The figure shows three views and two pictorial views of one solid part (mm, origin at its lowest corner). Answer the questions. A direction names the side the tool comes from. Round coordinates to 2 decimals unless told otherwise and drop trailing zeros. Write each loop counter-clockwise with the first axis right and the second up, starting at its lowest first coordinate (ties: lowest second). Pieces come first, ordered by that corner, then holes. Notation, with made-up numbers: (2, 83.25) - (20, 83.25) arc R26 cw to (20, 106.25) - close; hole circle Ø5 at (-39, 37.5). An arc over 180 degrees is marked (long way). Answer as CSV lines item,"result". Start each with the question number.
Item 1: A cutting plane is placed at C-C on y = 8. Determine the outline of the cut face in (x, z), and give its area (3 significant figures).
Item 2: A cutting plane is placed at D-D on x = 132.5. Determine the outline of the cut face in (y, z).
Item 3: Flat-ended cylindrical pins translate along their axes: pin 1 (6 mm diameter, centred on y = 11.5, z = 10, fed in from +X); pin 2 (9 mm diameter, centred on x = 10, y = 17.5, fed in from +Z); pin 3 (10.5 mm diameter, centred on x = 98.5, y = 23, fed in from -Z). Find the tip coordinate at first contact, or state that the pin passes through.
Item 4: A cutting plane is placed at B-B on z = 24. Determine the outline of the cut face in (x, y), and give its area (3 significant figures).
Item 5: A cutting plane is placed at A-A on x = 220. Determine the outline of the cut face in (y, z).
Item 6: For a pull along X with two mould halves and no side action, classify the marked faces 1, 2 and 3 as pulls with the +X half, pulls with the -X half, needs draft (parallel to the pull), parting line crosses it, or undercut.
Item 7: Which of the six approach directions +Z, -Z, +X, -X, +Y, -Y give full straight-line access (tool end or side, diameter ignored) to the marked faces 4 and 5?
Item 8: Straight lines are drawn through the part: line 1 along X through (y, z) = (27, 6.5); line 2 along Y through (x, z) = (147.5, 48.6); line 3 along Y through (x, z) = (10, 1.1). For each, find the intervals that lie inside material, in ascending order. Write a range as [from, to].
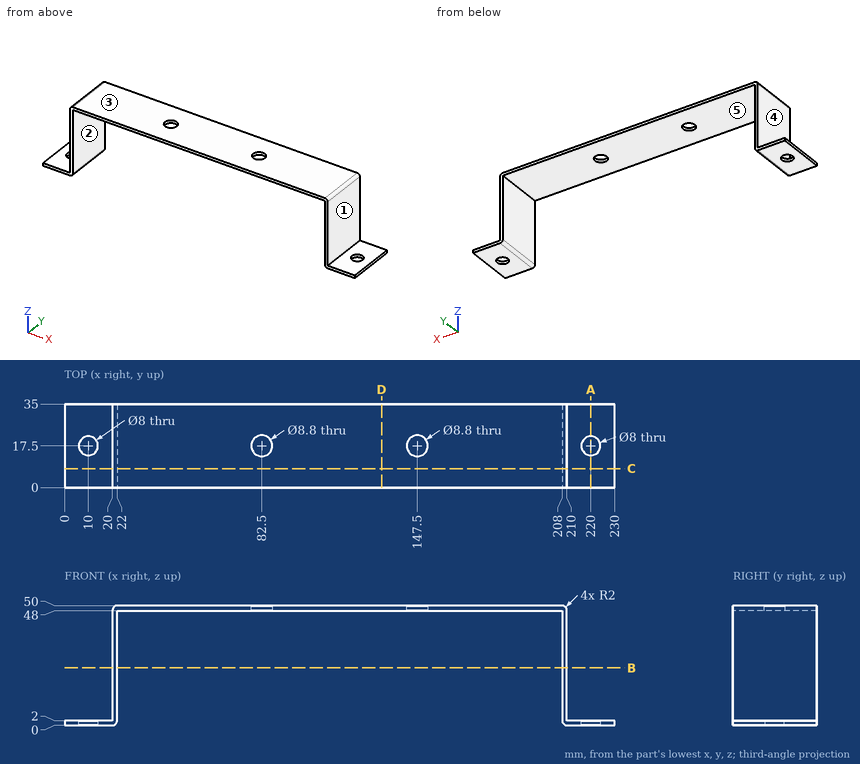
Geometry says:
1,outline,"(0, 0) - (20, 0) arc R2 ccw to (22, 2) - (22, 48) - (208, 48) - (208, 2) arc R2 ccw to (210, 0) - (230, 0) - (230, 2) - (210, 2) - (210, 48) arc R2 ccw to (208, 50) - (22, 50) arc R2 ccw to (20, 48) - (20, 2) - (0, 2) - close"
1,area,"649 mm^2"
2,outline,"(0, 48) - (35, 48) - (35, 50) - (0, 50) - close"
3,pin 1,"stops at x = 210"
3,pin 2,"stops at z = 2"
3,pin 3,"stops at z = 48"
4,outline,"(20, 0) - (22, 0) - (22, 35) - (20, 35) - close; (208, 0) - (210, 0) - (210, 35) - (208, 35) - close"
4,area,"140 mm^2"
5,outline,"(0, 0) - (13.5, 0) - (13.5, 2) - (0, 2) - close; (21.5, 0) - (35, 0) - (35, 2) - (21.5, 2) - close"
6,face 1,"pulls with the +X half"
6,face 2,"undercut"
6,face 3,"needs draft"
7,face 4,"+Z, -X, +Y, -Y"
7,face 5,"-Z, +Y, -Y"
8,line 1,"x = [20, 22], [208, 210]"
8,line 2,"y = [0, 13.1], [21.9, 35]"
8,line 3,"y = [0, 13.5], [21.5, 35]"
